from build123d import *

# Parameters (mm, degrees)
F0_W     = 23
F0_H     = 27
F0_W_2   = 19
F0_H_2   = 23
F1_DEPTH = 5
F3_DEPTH = 7
F5_DEPTH = 9


with BuildPart() as f1:
    # F0 (on Top) → F1 (new body)
    with BuildSketch(Plane.XY):
        with Locations((9.5, 11.5)):
            Rectangle(F0_W, F0_H)
        with Locations((9.5, 11.5)):
            Rectangle(F0_W_2, F0_H_2, mode=Mode.SUBTRACT)
    extrude(amount=F1_DEPTH)

    # F2 (on face) → F3 (join)
    with BuildSketch(Plane.XY.offset(5)):
        Polygon((3, 0), (0, 0), (0, 3), (-2, 3), (-2, -2), (3, -2), align=None)
    extrude(amount=F3_DEPTH)

    # F4 (on face) → F5 (join)
    with BuildSketch(Plane.XY.offset(5)):
        Polygon((19, 3), (19, 0), (16, 0), (16, -2), (21, -2), (21, 3), align=None)
    extrude(amount=F5_DEPTH)


solid = f1.part
Work out the finished part from the listing and answer in its coordinate system (mm). A direction names the side the tool comes from. Coordinates: 2 decimals unless noted, no trailing zeros. Loops run counter-clockwise (first coordinate to the right, second up) from the corner with the lowest first, then second, coordinate; pieces in that order, holes last. Notation, with made-up numbers: (33.5, 51.5) -> (52.5, 51.5) arc R6 cw to (52.5, 55.5) -> close; hole circle Ø4 at (5.25, 84). An arc over 180 degrees is marked (long way). Write each question's results on one line, items separated by ' | '. Start each with the question number.
1) The mould has two halves that part along Y. Classify faces 5 (the flat face through (20, 3, 9)), 6 (the flat face through (16, -1, 9)), 7 (the flat face through (19, 9, 4)): pulls with the +Y half, pulls with the -Y half, needs draft (parallel to the pull), parting line crosses it, or undercut.
2) Find section B-B on y = 10.5. Determine the outline of the cut face in (x, z), then the cut area to 3 significant figures.
3) Consider line 1 along Y through (x, z) = (1.5, 1); line 2 along X through (y, z) = (20.5, 3); line 3 along Z through (x, y) = (5, 23.75). Determine where each line is inside the solid, lowest interval first.
4) Flat-ended cylindrical pins translate along their axes: P1, Ø11, axis at x = 4, y = 16.5, coming from the +Z side; P2, Ø4, axis at x = -0.5, y = 0, coming from the +Z side; P3, Ø1.6, axis at x = 20, z = 11.5, coming from the +Y side. Find the tip coordinate at first contact, or state that the pin passes through.
5) Find section C-C on x = 9. Determine the outline of the cut face in (y, z), then the cut area to 3 significant figures.
6) For faces 1 (the flat face through (0, -1, 12)), 2 (the flat face through (3, -1, 8)), 3 (the flat face through (9, 23, 2)), 4 (the flat face through (-1, 3, 8)), determine the directions among +Z, -Z, +X, -X, +Y, -Y from which every point of the face is accessible in a straight line to the end or side of a thin tool.
7) Find section D-D on z = 1. Determine the outline of the cut face in (x, y).
8) Find section A-A on z = 10.5. Determine the outline of the cut face in (x, y).
Response values:
1) face 5: pulls with the +Y half | face 6: needs draft | face 7: undercut
2) outline: (-2, 0) -> (0, 0) -> (0, 5) -> (-2, 5) -> close; (19, 0) -> (21, 0) -> (21, 5) -> (19, 5) -> close | area: 20.0 mm^2
3) line 1: y = -2 to 0, 23 to 25 | line 2: x = -2 to 0, 19 to 21 | line 3: z = 0 to 5
4) P1: stops at z = 5 | P2: stops at z = 12 | P3: stops at y = 3
5) outline: (-2, 0) -> (0, 0) -> (0, 5) -> (-2, 5) -> close; (23, 0) -> (25, 0) -> (25, 5) -> (23, 5) -> close | area: 20.0 mm^2
6) face 1: +Z, -X, +Y, -Y | face 2: +Z, +Y, -Y | face 3: +Z, -Z | face 4: +Z, +X, -X, +Y
7) outline: (-2, -2) -> (21, -2) -> (21, 25) -> (-2, 25) -> close; hole (0, 0) -> (19, 0) -> (19, 23) -> (0, 23) -> close
8) outline: (-2, -2) -> (3, -2) -> (3, 0) -> (0, 0) -> (0, 3) -> (-2, 3) -> close; (16, -2) -> (21, -2) -> (21, 3) -> (19, 3) -> (19, 0) -> (16, 0) -> close
